Source: CAD feature listing. Evaluate the final solid. Frame: model axes, mm. A direction names the side the tool comes from. Round coordinates to 2 decimals unless told otherwise and drop trailing zeros. Order: outer loops, then holes, each group sorted by start corner. A loop starts at its lowest first (then second) coordinate and runs counter-clockwise, first axis right, second up. Notation, with made-up numbers: (33, 46) - (87, 46) arc R23 ccw to (87, 69) - close; hole circle Ø2 at (-18, -31). An arc over 180 degrees is marked (long way). Use one line per item in the form item = value. Start each with the question number.
Q1. Pin query (flat end, axial travel): pin 1 Ø5.5 at (x, y) = (-19.5, 0.5) entering from -Z (3 decimals); pin 2 Ø0.7 at (x, z) = (-13, 2) entering from -Y; pin 3 Ø1.5 at (y, z) = (4.5, 14.5) entering from +X; pin 4 Ø1.5 at (y, z) = (6, 41) entering from -X. Return the tip coordinate at first contact, or that it passes through.
Q2. Set-up query: faces 1 (the flat face through (-17.11, -1.2, 8.8)), 2 (the flat face through (-11, 2, 15.24)), 3 (the flat face through (-22, 1.479, 9)), 4 (the flat face through (-17, -2.09, 9)), 5 (the flat face through (-26.49, 2.35, 8.8)). Return all of +Z, -Z, +X, -X, +Y, -Y with unobstructed straight access to the full face (end or side cutting, diameter ignored); none if empty.
Q3. Cut plane A-A, the plane z = 42. Return the cut outline in (x, y), and give its area (3 significant figures).
Q4. Cut plane D-D, the plane z = 17. Return the cut outline in (x, y).
Q5. Cut plane C-C, the plane x = 0. Return the cut outline in (y, z).
Q6. Draft query along X for faces 6 (the flat face through (2.54, 0, 37)), 7 (the flat face through (-11, 1.479, 9)). Return one class per face: released by +X, released by -X, zero draft, split by the parting line, or undercut.
Q7. Ray query, line 1 (Z direction, x = -2.5, y = -5.25); line 2 (Z direction, x = -20.5, y = -1) (3 decimals); line 3 (X direction, y = -3, z = 36). Return the intervals inside material, ascending. Write a range as [from, to].
Q8. Cut plane B-B, the plane z = 5. Give the number of separate pieces and of enclosed holes in the cut face, and give its area (3 significant figures).
from build123d import *

# Parameters (mm, degrees)
F1_DEPTH = 48.26
F2_DEPTH = 25.4
F3_R     = 8.133276
F4_DEPTH = 2.54
F5_W     = 25.4
F5_H     = 6.734311
F6_DEPTH = 0.635
F8_DEPTH = 12.7


with BuildPart() as f1:
    # F0 (on Top) → F1 (new body)
    with BuildSketch(Plane.XY):
        with BuildLine():
            Line((-2.54, -2.805053), (-3.769917, -2.805053))
            ThreePointArc((-3.769917, -2.805053), (-0.00142, -4.699), (3.768222, -2.807331))
            Line((3.768222, -2.807331), (2.54, -2.807331))
            Line((2.54, -2.807331), (2.54, -2.667))
            ThreePointArc((2.54, -2.667), (0, -3.683), (-2.54, -2.667))
            Line((-2.54, -2.667), (-2.54, -2.805053))
        make_face()
        with BuildLine():
            Line((2.54, 0), (2.54, -2.667))
            ThreePointArc((2.54, -2.667), (3.385211, -1.450805), (3.683, 0))
            ThreePointArc((3.683, 0), (3.385211, 1.450805), (2.54, 2.667))
            Line((2.54, 2.667), (2.54, 0))
        make_face()
        with BuildLine():
            Line((2.54, -2.807331), (3.768222, -2.807331))
            Line((3.768222, -2.807331), (3.768222, 2.667))
            Line((3.768222, 2.667), (2.54, 2.667))
            ThreePointArc((2.54, 2.667), (3.385211, 1.450805), (3.683, 0))
            ThreePointArc((3.683, 0), (3.385211, -1.450805), (2.54, -2.667))
            Line((2.54, -2.667), (2.54, -2.807331))
        make_face()
        with BuildLine():
            ThreePointArc((3.768222, -2.807331), (4.46024, -1.478805), (4.699, 0))
            ThreePointArc((4.699, 0), (-1.477457, 4.460686), (-3.769917, -2.805053))
            Line((-3.769917, -2.805053), (-3.769917, 2.667))
            Line((-3.769917, 2.667), (-2.54, 2.667))
            ThreePointArc((-2.54, 2.667), (0, 3.683), (2.54, 2.667))
            Line((2.54, 2.667), (3.768222, 2.667))
            Line((3.768222, 2.667), (3.768222, -2.807331))
        make_face()
        with BuildLine():
            Line((-3.769917, 2.667), (-3.769917, -2.805053))
            Line((-3.769917, -2.805053), (-2.54, -2.805053))
            Line((-2.54, -2.805053), (-2.54, -2.667))
            ThreePointArc((-2.54, -2.667), (-3.683, 0), (-2.54, 2.667))
            Line((-2.54, 2.667), (-3.769917, 2.667))
        make_face()
        with BuildLine():
            ThreePointArc((-2.54, 2.667), (-3.683, 0), (-2.54, -2.667))
            Line((-2.54, -2.667), (-2.54, 0))
            Line((-2.54, 0), (-2.54, 2.667))
        make_face()
    extrude(amount=F1_DEPTH)

    # F0 (on Top) → F2 (join)
    with BuildSketch(Plane.XY):
        with BuildLine():
            Line((-2.54, 0), (-2.54, -2.667))
            ThreePointArc((-2.54, -2.667), (0, -3.683), (2.54, -2.667))
            Line((2.54, -2.667), (2.54, 0))
            Line((2.54, 0), (0, 0))
            Line((0, 0), (-2.54, 0))
        make_face()
        with BuildLine():
            ThreePointArc((2.54, 2.667), (0, 3.683), (-2.54, 2.667))
            Line((-2.54, 2.667), (-2.54, 0))
            Line((-2.54, 0), (0, 0))
            Line((0, 0), (2.54, 0))
            Line((2.54, 0), (2.54, 2.667))
        make_face()
    extrude(amount=F2_DEPTH)

    # F3 (on Top) → F4 (join)
    with BuildSketch(Plane.XY):
        Circle(F3_R)
    extrude(amount=F4_DEPTH)

    # F5 (on face) → F6 (join)
    with BuildSketch(Plane.XY.offset(2.54)):
        with Locations((-15.95207, 0.237246)):
            Rectangle(F5_W, F5_H)
    extrude(amount=-F6_DEPTH)

    # F7 (on face) → F8 (join)
    with BuildSketch(Plane.XY.offset(2.54)):
        Polygon((-27.00107, 3.238266), (-28.01707, 1.478502), (-25.98507, 1.478502), align=None)
        Polygon((-22.73387, 1.478502), (-20.70187, 1.478502), (-21.71787, 3.238266), align=None)
        Polygon((-17.45067, 1.478502), (-15.41867, 1.478502), (-16.43467, 3.238266), align=None)
        Polygon((-12.16747, 1.478502), (-10.13547, 1.478502), (-11.15147, 3.238266), align=None)
        Polygon((-27.174182, -0.329896), (-28.190182, -2.089659), (-26.158182, -2.089659), align=None)
        Polygon((-22.906982, -2.089659), (-20.874982, -2.089659), (-21.890982, -0.329896), align=None)
        Polygon((-17.623782, -2.089659), (-15.591782, -2.089659), (-16.607782, -0.329896), align=None)
        Polygon((-12.340582, -2.089659), (-10.308582, -2.089659), (-11.324582, -0.329896), align=None)
    extrude(amount=F8_DEPTH)


solid = f1.part
Completed:
q1.pin_1 = 1.905
q1.pin_2 = -3.13
q1.pin_3 = 2.83
q1.pin_4 = through
q2.face_1 = +Z
q2.face_2 = +Z, -X, +Y, -Y
q2.face_3 = +Z, -X
q2.face_4 = +Z, -X, -Y
q2.face_5 = +Z, +Y
q3.outline = (3.77, -2.81) arc R4.7 ccw to (4.7, 0) arc R4.7 ccw (long way) to start; hole (-2.54, -2.67) arc R3.68 ccw to (2.54, -2.67) - (2.54, 2.67) arc R3.68 ccw to (-2.54, 2.67) - close
q3.area = 35.2 mm2
q4.outline = (3.77, -2.81) arc R4.7 ccw to (4.7, 0) arc R4.7 ccw (long way) to start
q5.outline = (-8.13, 0) - (8.13, 0) - (8.13, 2.54) - (4.7, 2.54) - (4.7, 48.26) - (3.68, 48.26) - (3.68, 25.4) - (-3.68, 25.4) - (-3.68, 48.26) - (-4.7, 48.26) - (-4.7, 2.54) - (-8.13, 2.54) - close
q6.face_6 = undercut
q6.face_7 = zero draft
q7.line_1 = [0, 2.54]
q7.line_2 = [1.905, 2.54]
q7.line_3 = [-3.62, -2.14], [2.14, 3.62]
q8.separate_pieces = 9
q8.enclosed_holes = 0
q8.area = 83.7 mm2
